from build123d import *

# Parameters (mm, degrees)
F0_R        = 1.6
F1_DEPTH    = 2
F2_T1_DEPTH = 2
F2_T3_DEPTH = 27
F4_DEPTH    = 25


# Not quite as in the source:
# - a fillet or chamfer that OpenCascade refuses, or shapes differently, is made with other operations: its cross-section is extruded or revolved along the edge and cut away or added


with BuildPart() as f1:
    # F0 (on Top) → F1 (new body)
    with BuildSketch(Plane.XY):
        with BuildLine():
            add(Edge.make_bspline(
                [(-23.1606136078, -2.1185675411), (-22.1073400579, -3.5656171477), (-20.9766129337, -4.8945797394), (-19.7798663886, -6.1017373718)],
                knots=[0, 0, 0, 0, 0.0881031872, 0.0881031872, 0.0881031872, 0.0881031872], degree=3))
            ThreePointArc((-23.1606136078, -2.1185675411), (-23.8473189399, -0.1389116439), (-23.3153209852, 1.887804878))
            Line((-23.3153209852, 1.887804878), (-34.0653209852, -15.5674951767))
            ThreePointArc((-34.0653209852, -15.5674951767), (-32.887804878, -20.5206210399), (-27.9346790148, -19.3431049328))
            Line((-27.9346790148, -19.3431049328), (-19.7798663886, -6.1017373718))
        make_face()
        with Locations((-31, -17.4553000547)):
            Circle(F0_R, mode=Mode.SUBTRACT)
        with BuildLine():
            ThreePointArc((-23.3153209852, 1.887804878), (-23.8473189399, -0.1389116439), (-23.1606136078, -2.1185675411))
            add(Edge.make_bspline(
                [(-23.1606136078, -2.1185675411), (-22.1073400579, -3.5656171477), (-20.9766129337, -4.8945797394), (-19.7798663886, -6.1017373718)],
                knots=[0, 0, 0, 0, 0.0881031872, 0.0881031872, 0.0881031872, 0.0881031872], degree=3))
            Line((-19.7798663886, -6.1017373718), (-17.1846790148, -1.887804878))
            ThreePointArc((-17.1846790148, -1.887804878), (-16.6526810601, 0.1389116439), (-17.3393863922, 2.1185675411))
            ThreePointArc((-17.3393863922, 2.1185675411), (-20.3889116439, 3.5973189399), (-23.3153209852, 1.887804878))
        make_face()
        with Locations((-20.25, 0)):
            Circle(F0_R, mode=Mode.SUBTRACT)
        with BuildLine():
            Line((-17.1846790148, -1.887804878), (-19.7798663886, -6.1017373718))
            add(Edge.make_bspline(
                [(-19.7798663886, -6.1017373718), (-19.2786798287, -6.6072840002), (-17.0287540912, -8.7317983569), (-12.6752714432, -11.7584634521), (-6.4699511651, -14.1622363484), (0, -14.9688818258), (6.4699511651, -14.1622363484), (12.6752714432, -11.7584634521), (17.0287540912, -8.7317983569), (19.2786798287, -6.6072840002), (19.7798663886, -6.1017373718)],
                knots=[0.0881031872, 0.0881031872, 0.0881031872, 0.0881031872, 0.125, 0.25, 0.375, 0.5, 0.625, 0.75, 0.875, 0.9118968128, 0.9118968128, 0.9118968128, 0.9118968128], degree=3))
            Line((19.7798663886, -6.1017373718), (17.1846790148, -1.887804878))
            ThreePointArc((17.1846790148, -1.887804878), (16.6526810601, 0.1389116439), (17.3393863922, 2.1185675411))
            add(Edge.make_bspline(
                [(-17.3393863922, 2.1185675411), (-16.1406178919, 0.4716283513), (-13.5435115335, -2.372660701), (-9.2367539572, -5.3540365479), (-4.6778336966, -7.1127636516), (0, -7.6936181742), (4.6778336966, -7.1127636516), (9.2367539572, -5.3540365479), (13.5435115335, -2.372660701), (16.1406178919, 0.4716283513), (17.3393863922, 2.1185675411)],
                knots=[0, 0, 0, 0, 0.125, 0.25, 0.375, 0.5, 0.625, 0.75, 0.875, 1, 1, 1, 1], degree=3))
            ThreePointArc((-17.3393863922, 2.1185675411), (-16.6526810601, 0.1389116439), (-17.1846790148, -1.887804878))
        make_face()
        with BuildLine():
            add(Edge.make_bspline(
                [(-19.7798663886, -6.1017373718), (-19.2786798287, -6.6072840002), (-17.0287540912, -8.7317983569), (-12.6752714432, -11.7584634521), (-6.4699511651, -14.1622363484), (0, -14.9688818258), (6.4699511651, -14.1622363484), (12.6752714432, -11.7584634521), (17.0287540912, -8.7317983569), (19.2786798287, -6.6072840002), (19.7798663886, -6.1017373718)],
                knots=[0.0881031872, 0.0881031872, 0.0881031872, 0.0881031872, 0.125, 0.25, 0.375, 0.5, 0.625, 0.75, 0.875, 0.9118968128, 0.9118968128, 0.9118968128, 0.9118968128], degree=3))
            Line((-19.7798663886, -6.1017373718), (-27.9346790148, -19.3431049328))
            Line((-27.9346790148, -19.3431049328), (-25, -19.3431049328))
            Line((-25, -19.3431049328), (-25, -40.5))
            Line((-25, -40.5), (0, -40.5))
            Line((0, -40.5), (25, -40.5))
            Line((25, -40.5), (25, -19.3431049328))
            Line((25, -19.3431049328), (27.9346790148, -19.3431049328))
            Line((27.9346790148, -19.3431049328), (19.7798663886, -6.1017373718))
        make_face()
        with BuildLine():
            Line((17.1846790148, -1.887804878), (19.7798663886, -6.1017373718))
            add(Edge.make_bspline(
                [(19.7798663886, -6.1017373718), (20.9766129337, -4.8945797394), (22.1073400579, -3.5656171477), (23.1606136078, -2.1185675411)],
                knots=[0.9118968128, 0.9118968128, 0.9118968128, 0.9118968128, 1, 1, 1, 1], degree=3))
            ThreePointArc((23.1606136078, -2.1185675411), (23.8473189399, -0.1389116439), (23.3153209852, 1.887804878))
            ThreePointArc((23.3153209852, 1.887804878), (20.3889116439, 3.5973189399), (17.3393863922, 2.1185675411))
            ThreePointArc((17.3393863922, 2.1185675411), (16.6526810601, 0.1389116439), (17.1846790148, -1.887804878))
        make_face()
        with Locations((20.25, 0)):
            Circle(F0_R, mode=Mode.SUBTRACT)
        with BuildLine():
            add(Edge.make_bspline(
                [(19.7798663886, -6.1017373718), (20.9766129337, -4.8945797394), (22.1073400579, -3.5656171477), (23.1606136078, -2.1185675411)],
                knots=[0.9118968128, 0.9118968128, 0.9118968128, 0.9118968128, 1, 1, 1, 1], degree=3))
            Line((19.7798663886, -6.1017373718), (27.9346790148, -19.3431049328))
            ThreePointArc((27.9346790148, -19.3431049328), (32.887804878, -20.5206210399), (34.0653209852, -15.5674951767))
            Line((34.0653209852, -15.5674951767), (23.3153209852, 1.887804878))
            ThreePointArc((23.3153209852, 1.887804878), (23.8473189399, -0.1389116439), (23.1606136078, -2.1185675411))
        make_face()
        with Locations((31, -17.4553000547)):
            Circle(F0_R, mode=Mode.SUBTRACT)
    extrude(amount=F1_DEPTH)

    # F2: fillet of radius 5 on 6 edges, made by hand

    # F2_s2 → F2_t1 (join)
    with BuildSketch(Plane.XY):
        with BuildLine():
            ThreePointArc((-25, -24.3431049328), (-26.4644660941, -20.8075710268), (-30, -19.3431049328))
            Line((-30, -19.3431049328), (-25, -19.3431049328))
            Line((-25, -19.3431049328), (-25, -24.3431049328))
        make_face()
        with BuildLine():
            ThreePointArc((-25.8504229337, -19.3431049328), (-27.4279703024, -19.598492799), (-28.8443630885, -20.338567213))
            ThreePointArc((-28.8443630885, -20.338567213), (-28.3424942846, -19.8838105802), (-27.9346790148, -19.3431049328))
            Line((-27.9346790148, -19.3431049328), (-25.8504229337, -19.3431049328))
        make_face()
        with BuildLine():
            ThreePointArc((30, -19.3431049328), (26.4644660941, -20.8075710268), (25, -24.3431049328))
            Line((25, -24.3431049328), (25, -19.3431049328))
            Line((25, -19.3431049328), (30, -19.3431049328))
        make_face()
        with BuildLine():
            ThreePointArc((28.8443630885, -20.338567213), (27.4279703024, -19.598492799), (25.8504229337, -19.3431049328))
            Line((25.8504229337, -19.3431049328), (27.9346790148, -19.3431049328))
            ThreePointArc((27.9346790148, -19.3431049328), (28.3424942846, -19.8838105802), (28.8443630885, -20.338567213))
        make_face()
    extrude(amount=F2_T1_DEPTH)

    # F2_s4 → F2_t3 (cut)
    with BuildSketch(Plane.XY.offset(-12.5)):
        with BuildLine():
            ThreePointArc((-25, -35.5), (-23.5355339059, -39.0355339059), (-20, -40.5))
            Line((-20, -40.5), (-25, -40.5))
            Line((-25, -40.5), (-25, -35.5))
        make_face()
        with BuildLine():
            ThreePointArc((20, -40.5), (23.5355339059, -39.0355339059), (25, -35.5))
            Line((25, -35.5), (25, -40.5))
            Line((25, -40.5), (20, -40.5))
        make_face()
    extrude(amount=F2_T3_DEPTH, mode=Mode.SUBTRACT)

    # F3 (on face) → F4 (cut)
    with BuildSketch(Plane.XY.offset(2)):
        with BuildLine():
            ThreePointArc((-17.5, -10.5), (-19, -12), (-17.5, -13.5))
            Line((-17.5, -13.5), (17.5, -13.5))
            ThreePointArc((17.5, -13.5), (19, -12), (17.5, -10.5))
            Line((17.5, -10.5), (-17.5, -10.5))
        make_face()
        with BuildLine():
            ThreePointArc((-17.5, -17.5), (-19, -19), (-17.5, -20.5))
            Line((-17.5, -20.5), (17.5, -20.5))
            ThreePointArc((17.5, -20.5), (19, -19), (17.5, -17.5))
            Line((17.5, -17.5), (-17.5, -17.5))
        make_face()
        with BuildLine():
            ThreePointArc((-17.5, -24.5), (-19, -26), (-17.5, -27.5))
            Line((-17.5, -27.5), (17.5, -27.5))
            ThreePointArc((17.5, -27.5), (19, -26), (17.5, -24.5))
            Line((17.5, -24.5), (-17.5, -24.5))
        make_face()
        with BuildLine():
            ThreePointArc((-17.5, -31.5), (-19, -33), (-17.5, -34.5))
            Line((-17.5, -34.5), (17.5, -34.5))
            ThreePointArc((17.5, -34.5), (19, -33), (17.5, -31.5))
            Line((17.5, -31.5), (-17.5, -31.5))
        make_face()
    extrude(amount=-F4_DEPTH, mode=Mode.SUBTRACT)


solid = f1.part
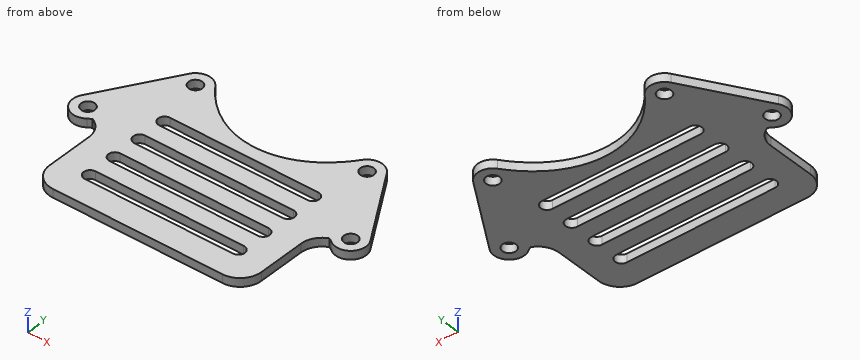
The model under review builds one solid part; all positions refer to its coordinate system, in mm. Give positions to 0.01 mm unless a question says otherwise; leave off trailing zeros. Loops run counter-clockwise (first coordinate to the right, second up) from the corner with the lowest first, then second, coordinate; pieces in that order, holes last. Notation, with made-up numbers: (-40, -12.75) -> (-31, -12.75) arc R23 ccw to (-31, 6.25) -> close; hole circle Ø4 at (-1, 67). An arc over 180 degrees is marked (long way). Write each question's results on one line, items separated by ' | '.
1) Take a section at A-A, the plane y = -33. Give the boundary of the cut face in (x, z), plus the area to 3 significant figures.
Conclusion:
outline: (-25, 0) -> (-19, 0) -> (-19, 2) -> (-25, 2) -> close; (19, 0) -> (25, 0) -> (25, 2) -> (19, 2) -> close | area: 24.0 mm^2
2) Take a section at B-B, the plane x = 31. Give the boundary of the cut face in (y, z), plus the area to 3 significant figures.
Conclusion:
outline: (-21.06, 0) -> (-19.06, 0) -> (-19.06, 2) -> (-21.06, 2) -> close; (-15.86, 0) -> (-10.59, 0) -> (-10.59, 2) -> (-15.86, 2) -> close | area: 14.5 mm^2
3) For line 1 along X through (y, z) = (-18, 1.3); line 2 along Y through (x, z) = (-11, 1.75); line 3 along Y through (x, z) = (-20.25, 1.4), list the stretches that pass through material, from the lowest coordinate up. Write a range as from..to.
Conclusion:
line 1: x = -34.56..-32.5, -29.5..-18.62, 18.62..29.5, 32.5..34.56 | line 2: y = -40.5..-34.5, -31.5..-27.5, -24.5..-20.5, -17.5..-13.5, -10.5..-4.07 | line 3: y = -40.49..-1.6, 1.6..3.6
4) Insertion check: pin 1 Ø1 at (y, z) = (-32, 0.5) entering from +X; pin 2 Ø3 at (x, y) = (20.25, 0) entering from -Z; pin 3 Ø0.6 at (x, z) = (-5, 1) entering from +Y; pin 4 Ø1 at (x, z) = (3, 1) entering from +Y. Each pin has a flat end and moves straight along its axis. Give the tip position at first contact, or say it passes through.
Conclusion:
pin 1: stops at x = 25 | pin 2: passes through | pin 3: stops at y = -6.74 | pin 4: stops at y = -7.17
5) Take a section at C-C, the plane x = 7.5. Count the separate pieces of the cut face and the enclosed holes in it, plus the area to 3 significant figures.
Conclusion:
separate pieces: 5 | enclosed holes: 0 | area: 45.1 mm^2
